Read the model definition and answer for the solid it produces. Units are mm, in the model's axes. A direction names the side the tool comes from. Give positions to 0.01 mm unless a question says otherwise; leave off trailing zeros. Write each loop counter-clockwise with the first axis right and the second up, starting at its lowest first coordinate (ties: lowest second). Pieces come first, ordered by that corner, then holes. Notation, with made-up numbers: (18, 28) -> (28, 28) arc R19 cw to (28, 47) -> close; hole circle Ø2 at (72, 82). An arc over 180 degrees is marked (long way). Write item = value, one per line.
from build123d import *

# Parameters (mm, degrees)
SKETCH_1_R          = 5
EXTRUDE_1_DEPTH     = 48
SKETCH_2_R          = 6
EXTRUDE_2_DEPTH     = 3
SKETCH_3_R          = 5
EXTRUDE_3_DEPTH     = 7
SKETCH_5_R          = 4
EXTRUDE_4_DEPTH     = 10
SKETCH_6_R          = 1.25
CUT_EXTRUDE_1_DEPTH = 10
CUT_EXTRUDE_START   = -10
SKETCH_7_R          = 1.25
CUT_EXTRUDE_2_DEPTH = 10


with BuildPart() as part:
    # 草图1 → 凸台-拉伸1 (new body)
    with BuildSketch(Plane.XY):
        Circle(SKETCH_1_R)
    extrude(amount=EXTRUDE_1_DEPTH)

    # 草图2 → 凸台-拉伸2 (add)
    with BuildSketch(Plane.XY.offset(48)):
        Circle(SKETCH_2_R)
    extrude(amount=EXTRUDE_2_DEPTH)

    # 草图3 → 凸台-拉伸3 (add)
    with BuildSketch(Plane.XY.offset(51)):
        Circle(SKETCH_3_R)
    extrude(amount=EXTRUDE_3_DEPTH)

    # 草图5 → 凸台-拉伸4 (add)
    with BuildSketch(Plane(origin=(0, 0, 0), x_dir=(-1, 0, 0), z_dir=(0, 0, -1))):
        Circle(SKETCH_5_R)
    extrude(amount=EXTRUDE_4_DEPTH)

    # 草图6 → 切除-拉伸1 (cut)
    with BuildSketch(Plane.XY.offset(58)):
        Circle(SKETCH_6_R)
    extrude(amount=-CUT_EXTRUDE_1_DEPTH, mode=Mode.SUBTRACT)

    # 草图7 → 切除-拉伸2 (cut)
    with BuildSketch(Plane(origin=(0, 0, -10), x_dir=(-1, 0, 0), z_dir=(0, 0, -1)).offset(CUT_EXTRUDE_START)):
        with Locations(Location((0, 0, 0), (0, 0, 180))):
            Circle(SKETCH_7_R)
    extrude(amount=CUT_EXTRUDE_2_DEPTH, mode=Mode.SUBTRACT)


solid = part.part
(1) The part is cut by section A-A on x = 0. Determine the outline of the cut face in (y, z).
Checks:
outline = (-6, 48) -> (-5, 48) -> (-5, 0) -> (-4, 0) -> (-4, -10) -> (-1.25, -10) -> (-1.25, 0) -> (1.25, 0) -> (1.25, -10) -> (4, -10) -> (4, 0) -> (5, 0) -> (5, 48) -> (6, 48) -> (6, 51) -> (5, 51) -> (5, 58) -> (1.25, 58) -> (1.25, 48) -> (-1.25, 48) -> (-1.25, 58) -> (-5, 58) -> (-5, 51) -> (-6, 51) -> close
(2) For a pull along Y with two mould halves and no side action, classify faces 4 (the cylindrical face through (-1.25, -0.05, -4.93)), 5 (the flat face through (0, 0, 0)), 6 (the flat face through (-4, 4, 51)), 7 (the cylindrical face through (-6, 0, 49)) as released by +Y, released by -Y, zero draft, split by the parting line, or undercut.
Checks:
face_4 = undercut
face_5 = undercut
face_6 = zero draft
face_7 = split by the parting line
(3) A tool of negligible diameter and unlimited length cuts with its end or side. For faces 1 (the cylindrical face through (0.867, -3.905, -4.93)), 2 (the cylindrical face through (-1.08, -4.88, 54.45)), 3 (the flat face through (1, -1, 58)), from which of +Z, -Z, +X, -X, +Y, -Y can it reach the whole face along a straight path? Write none if from no direction.
Checks:
face_1 = -Z
face_2 = +Z
face_3 = +Z, +X, -X, +Y, -Y
(4) The part is cut by section D-D on y = 3. Determine the outline of the cut face in (x, z).
Checks:
outline = (-5.2, 48) -> (-4, 48) -> (-4, 0) -> (-2.65, 0) -> (-2.65, -10) -> (2.65, -10) -> (2.65, 0) -> (4, 0) -> (4, 48) -> (5.2, 48) -> (5.2, 51) -> (4, 51) -> (4, 58) -> (-4, 58) -> (-4, 51) -> (-5.2, 51) -> close
(5) The part is cut by section C-C on x = 2.5. Determine the outline of the cut face in (y, z), plus the area to 3 significant figures.
Checks:
outline = (-5.45, 48) -> (-4.33, 48) -> (-4.33, 0) -> (-3.12, 0) -> (-3.12, -10) -> (3.12, -10) -> (3.12, 0) -> (4.33, 0) -> (4.33, 48) -> (5.45, 48) -> (5.45, 51) -> (4.33, 51) -> (4.33, 58) -> (-4.33, 58) -> (-4.33, 51) -> (-5.45, 51) -> close
area = 571 mm²
(6) Consider L1, parallel to Y at x = 0, z = 51.5; L2, parallel to Z at x = -3.5, y = -4; L3, parallel to Z at x = -3.75, y = -1.5. Determine where each line is inside the solid, lowest interval first.
Checks:
L1 = -5 to -1.25, 1.25 to 5
L2 = 48 to 51
L3 = 0 to 58
(7) Given P1, Ø2, axis at x = 4.5, z = 44, coming from the -Y side; P2, Ø5, axis at x = -0.5, y = 0, coming from the -Z side; P3, Ø0.8, axis at x = 0, y = -0.5, coming from the -Z side; P4, Ø2, axis at y = 1.5, z = 13, coming from the +X side, each flat-ended and moving along its own axis, determine where each tip first touches the part or whether it passes through.
Checks:
P1 = -3.57
P2 = -10
P3 = 0
P4 = 4.97
